Work out the finished part from the listing and answer in its coordinate system (mm). Give positions to 0.01 mm unless a question says otherwise; leave off trailing zeros. Loops run counter-clockwise (first coordinate to the right, second up) from the corner with the lowest first, then second, coordinate; pieces in that order, holes last. Notation, with made-up numbers: (-3, 14.25) - (40, 14.25) arc R22 cw to (40, 26.25) - close; hole circle Ø5 at (49, 4). An arc over 180 degrees is marked (long way). One line per question, with ' | ' between items. Start each with the question number.
1. This flat-tipped pin is pushed along its axis until it touches: pin 1 (1.5 mm diameter, centred on x = -0.5, y = 0, fed in from -Z). Where does it stop, or does it pass through?
2. For a pull along X with two mould halves and no side action, classify faces 1 (the face through (2.278, -0.796, 0.003)), 2 (the face through (-0.115, -3.173, 0.003)), 3 (the face through (0, -2, -0.19)), 4 (the face through (-2.29, -0.76, 0)) as released by +X, released by -X, zero draft, split by the parting line, or undercut.
3. Section D-D (y = -1.65) is taken. Determine the outline of the cut face in (x, z), plus the area to 3 significant figures.
4. Section C-C (x = -1.5) is taken. Determine the outline of the cut face in (y, z), plus the area to 3 significant figures.
5. Find the intervals of material crossed by line 1 (X direction, y = -0.1, z = -0.05); line 2 (X direction, y = 1.4, z = -0.05); line 3 (Y direction, x = 0, z = -0.1) (3 decimals), in increasing order.
6. Section B-B (z = 0.1) is taken. Determine the outline of the cut face in (x, y) (3 decimals).
from build123d import *
from OCP.BRepFilletAPI import BRepFilletAPI_MakeFillet

# Parameters (mm, degrees)
SKETCH1_R           = 3.175
SKETCH1_R_2         = 1.190625
BOSS_EXTRUDE1_DEPTH = 0.1905
CUT_EXTRUDE1_DEPTH  = 5.50626353
CUT_EXTRUDE2_DEPTH  = 5.50626353
FILLET1_R1          = 0.381
FILLET1_R2          = 0.127


with BuildPart() as part:
    # Sketch1 → Boss-Extrude1 (new, symmetric)
    with BuildSketch(Plane.XY):
        with Locations(Location((0, 0, 0), (0, 0, 180))):
            Circle(SKETCH1_R)
        with Locations(Location((0, 0, 0), (0, 0, 180))):
            Circle(SKETCH1_R_2, mode=Mode.SUBTRACT)
    extrude(amount=BOSS_EXTRUDE1_DEPTH, both=True)

    # Sketch2 → Cut-Extrude1 (cut, through all)
    with BuildSketch(Plane.XY.offset(0.1905)):
        Polygon((-0.635, 0.3107001), (0.635, 0.3107001), (1.27, 3.175), (-1.27, 3.175), align=None)
    extrude(amount=-CUT_EXTRUDE1_DEPTH, mode=Mode.SUBTRACT)

    # Sketch3 → Cut-Extrude2 (cut, through all)
    with BuildSketch(Plane.XY.offset(0.1905)):
        with BuildLine():
            Line((-1.05664, 0.548725615), (-2.140900128, 1.113155712))
            ThreePointArc((-2.140900128, 1.113155712), (-2.284707131, -0.776326171), (-1.019518005, -2.187041846))
            Line((-1.019518005, -2.187041846), (-0.50292, -1.079193849))
            ThreePointArc((-0.50292, -1.079193849), (-1.127203307, -0.383406568), (-1.05664, 0.548725615))
        make_face()
        with BuildLine():
            Line((0.50292, -1.079193849), (1.019518005, -2.187041846))
            ThreePointArc((1.019518005, -2.187041846), (2.284707131, -0.776326171), (2.140900128, 1.113155712))
            Line((2.140900128, 1.113155712), (1.05664, 0.548725615))
            ThreePointArc((1.05664, 0.548725615), (1.127203307, -0.383406568), (0.50292, -1.079193849))
        make_face()
    extrude(amount=-CUT_EXTRUDE2_DEPTH, mode=Mode.SUBTRACT)

    # Fillet1: one fillet with a radius per group of edges: ONE call of the kernel's fillet builder (fillet() takes one radius for all edges)
    fillet1_edges_1 = [part.edges().sort_by_distance(p)[0] for p in [
        (-1.216302436, 2.932785942, 0),
        (-2.140900128, 1.113155712, 0),
        (-1.019518005, -2.187041846, 0),
        (1.019518005, -2.187041846, 0),
        (2.140900128, 1.113155712, 0),
        (1.216302436, 2.932785942, 0),
    ]]
    fillet1_edges_2 = [part.edges().sort_by_distance(p)[0] for p in [
        (-0.767848913, 0.909942821, 0),
        (-1.05664, 0.548725615, 0),
        (0.767848913, 0.909942821, 0),
        (1.05664, 0.548725615, 0),
    ]]
    fillet1 = BRepFilletAPI_MakeFillet(part.part.solid().wrapped)
    for e in fillet1_edges_1:
        fillet1.Add(FILLET1_R1, e.wrapped)
    for e in fillet1_edges_2:
        fillet1.Add(FILLET1_R2, e.wrapped)
    add(Compound.cast(fillet1.Shape()), mode=Mode.REPLACE)


solid = part.part
Conclusion:
1) pin 1: through
2) face 1: undercut | face 2: split by the parting line | face 3: zero draft | face 4: undercut
3) outline: (-2.71, -0.19) - (-1.76, -0.19) - (-1.76, 0.19) - (-2.71, 0.19) - close; (-0.77, -0.19) - (0.77, -0.19) - (0.77, 0.19) - (-0.77, 0.19) - close; (1.76, -0.19) - (2.71, -0.19) - (2.71, 0.19) - (1.76, 0.19) - close | area: 1.31 mm²
4) outline: (-2.8, -0.19) - (-1.89, -0.19) - (-1.89, 0.19) - (-2.8, 0.19) - close; (0.78, -0.19) - (2.75, -0.19) - (2.75, 0.19) - (0.78, 0.19) - close | area: 1.10 mm²
5) line 1: -3.17 to -2.41, 2.41 to 3.17 | line 2: -2.85 to -0.88, 0.88 to 2.85 | line 3: -3.175 to -1.191
6) outline: (-2.312, 0.692) arc R0.381 cw to (-1.771, 0.92) - (-1.164, 0.605) arc R0.127 ccw to (-0.999, 0.648) arc R1.191 cw to (-0.82, 0.863) arc R0.127 ccw to (-0.784, 0.982) - (-1.11, 2.451) arc R0.381 ccw to (-1.684, 2.692) arc R3.175 ccw (long way) to (1.684, 2.692) arc R0.381 ccw to (1.11, 2.451) - (0.784, 0.982) arc R0.127 ccw to (0.82, 0.863) arc R1.191 cw to (0.999, 0.648) arc R0.127 ccw to (1.164, 0.605) - (1.771, 0.92) arc R0.381 cw to (2.312, 0.692) arc R2.413 cw to (1.411, -1.957) arc R0.381 cw to (0.843, -1.809) - (0.503, -1.079) arc R1.191 cw to (-0.503, -1.079) - (-0.843, -1.809) arc R0.381 cw to (-1.411, -1.957) arc R2.413 cw to start
